CAD build for the part. Positions are in the model's coordinates, mm. Face numbers are marked on the shaded views. A direction names the side the tool comes from. Coordinates: 2 decimals unless noted, no trailing zeros. Order: outer loops, then holes, each group sorted by start corner. A loop starts at its lowest first (then second) coordinate and runs counter-clockwise, first axis right, second up. Notation, with made-up numbers: M -22.75,77.25 L 23.25,77.25 A16 ccw 23.25,87.25 Z; hole C 69,73 d1. An arc over 180 degrees is marked long. One line per item, written item: value.
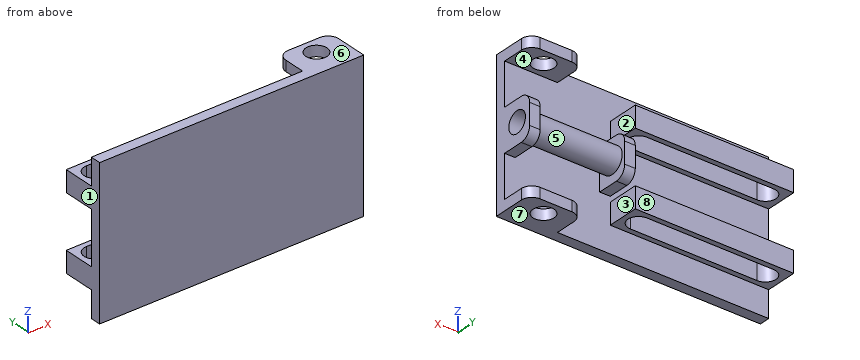
from build123d import *

# Parameters (mm, degrees)
SKETCH1_W           = 250
SKETCH1_H           = 140
BOSS_EXTRUDE1_DEPTH = 10
SKETCH2_W           = 150
SKETCH2_H           = 20
SKETCH2_W_2         = 50
BOSS_EXTRUDE2_DEPTH = 30
CUT_EXTRUDE1_DEPTH  = 120
SKETCH4_R           = 10
CUT_EXTRUDE2_DEPTH  = 150
SKETCH6_W           = 10
SKETCH6_H           = 40
CUT_EXTRUDE4_DEPTH  = 150
SKETCH7_R           = 10
CUT_EXTRUDE5_DEPTH  = 150
SKETCH8_R           = 12
SKETCH8_R_2         = 10
BOSS_EXTRUDE3_DEPTH = 80
SKETCH9_W           = 40
SKETCH9_H           = 30
SKETCH9_R           = 10
BOSS_EXTRUDE4_DEPTH = 10
FILLET1_R           = 10
FILLET2_R           = 10
FILLET3_R           = 10
SKETCH13_W          = 50
SKETCH13_H          = 25
SKETCH13_H_2        = 22.244291656
CUT_EXTRUDE6_DEPTH  = 40


with BuildPart() as part:
    # Sketch1 → Boss-Extrude1 (new body)
    with BuildSketch(Plane(origin=(0, 0, 0), x_dir=(1, 0, 0), z_dir=(0, 1, 0))):
        Rectangle(SKETCH1_W, SKETCH1_H)
    extrude(amount=BOSS_EXTRUDE1_DEPTH)

    # Sketch2 → Boss-Extrude2 (add)
    with BuildSketch(Plane(origin=(0, 10, 0), x_dir=(1, 0, 0), z_dir=(0, 1, 0))):
        with Locations((-50, 35)):
            Rectangle(SKETCH2_W, SKETCH2_H)
        with Locations((-50, -35)):
            Rectangle(SKETCH2_W, SKETCH2_H)
        Polygon((125, -20), (125, 0), (125, 20), (105, 20), (105, -20), align=None)
        with Locations((100, 60)):
            Rectangle(SKETCH2_W_2, SKETCH2_H)
        with Locations((100, -60)):
            Rectangle(SKETCH2_W_2, SKETCH2_H)
    extrude(amount=BOSS_EXTRUDE2_DEPTH)

    # Sketch3 → Cut-Extrude1 (cut)
    with BuildSketch(Plane.XY.offset(45)):
        with BuildLine():
            Line((10, 35), (-110, 35))
            ThreePointArc((-110, 35), (-120, 25), (-110, 15))
            Line((-110, 15), (10, 15))
            ThreePointArc((10, 15), (20, 25), (10, 35))
        make_face()
    extrude(amount=-CUT_EXTRUDE1_DEPTH, mode=Mode.SUBTRACT)

    # Sketch4 → Cut-Extrude2 (cut)
    with BuildSketch(Plane.XY.offset(70)):
        with Locations((100, 25)):
            Circle(SKETCH4_R)
    extrude(amount=-CUT_EXTRUDE2_DEPTH, mode=Mode.SUBTRACT)

    # Sketch6 → Cut-Extrude4 (cut)
    with BuildSketch(Plane(origin=(0, 10, 0), x_dir=(1, 0, 0), z_dir=(0, 1, 0))):
        with Locations((110, 0)):
            Rectangle(SKETCH6_W, SKETCH6_H)
    extrude(amount=CUT_EXTRUDE4_DEPTH, mode=Mode.SUBTRACT)

    # Sketch7 → Cut-Extrude5 (cut)
    with BuildSketch(Plane(origin=(125, 0, 0), x_dir=(0, 0, -1), z_dir=(1, 0, 0))):
        with Locations((0, 25)):
            Circle(SKETCH7_R)
    extrude(amount=-CUT_EXTRUDE5_DEPTH, mode=Mode.SUBTRACT)

    # Sketch8 → Boss-Extrude3 (add)
    with BuildSketch(Plane.ZY.offset(-115)):
        with Locations((0, 25)):
            Circle(SKETCH8_R)
        with Locations(Location((0, 25, 0), (0, 0, 180))):
            Circle(SKETCH8_R_2, mode=Mode.SUBTRACT)
    extrude(amount=BOSS_EXTRUDE3_DEPTH)

    # Sketch9 → Boss-Extrude4 (add)
    with BuildSketch(Plane.ZY.offset(-35)):
        with Locations((0, 25)):
            Rectangle(SKETCH9_W, SKETCH9_H)
        with Locations(Location((0, 25, 0), (0, 0, 180))):
            Circle(SKETCH9_R, mode=Mode.SUBTRACT)
    extrude(amount=BOSS_EXTRUDE4_DEPTH)

    # Fillet1
    fillet1_edges = [part.edges().sort_by_distance(p)[0] for p in [
        (30, 40, 20),
        (30, 40, -20),
    ]]
    fillet(fillet1_edges, radius=FILLET1_R)

    # Fillet2
    fillet2_edges = [part.edges().sort_by_distance(p)[0] for p in [
        (120, 40, 20),
        (120, 40, -20),
    ]]
    fillet(fillet2_edges, radius=FILLET2_R)

    # Fillet3
    fillet3_edges = [part.edges().sort_by_distance(p)[0] for p in [
        (75, 40, -60),
        (125, 40, -60),
        (75, 40, 60),
        (125, 40, 60),
    ]]
    fillet(fillet3_edges, radius=FILLET3_R)

    # Sketch13 → Cut-Extrude6 (cut)
    with BuildSketch(Plane(origin=(0, 10, 0), x_dir=(1, 0, 0), z_dir=(0, 1, 0))):
        with Locations((100, 47.5)):
            Rectangle(SKETCH13_W, SKETCH13_H)
        with Locations((100, -48.877854172)):
            Rectangle(SKETCH13_W, SKETCH13_H_2)
    extrude(amount=CUT_EXTRUDE6_DEPTH, mode=Mode.SUBTRACT)


solid = part.part
Q1. Slice it at D-D (y = 25). Give the number of separate pieces and of enclosed holes in the cut face, plus the area to 3 significant figures.
Recorded:
separate pieces: 10
enclosed holes: 0
area: 1,720 mm^2
Q2. Pin check, flat tips, straight feed: pin 1 Ø8 at (y, z) = (19.5, -65.5) entering from -X; pin 2 Ø8 at (x, z) = (-32, -3.5) entering from +Y; pin 3 Ø16 at (y, z) = (25, -35) entering from +X; pin 4 Ø9 at (x, y) = (-62.5, 22) entering from -Z. Stop position of each tip, or through.
Recorded:
pin 1: stops at x = 75
pin 2: stops at y = 10
pin 3: stops at x = 25
pin 4: passes through
Q3. Slice it at C-C (x = -100.5). List the corners of the cut face in (y, z), plus the area to 3 significant figures.
Recorded:
outline: M 0,-70 L 10,-70 L 10,-45 L 15,-45 L 15,-25 L 10,-25 L 10,25 L 15,25 L 15,45 L 10,45 L 10,70 L 0,70 Z; M 35,-45 L 40,-45 L 40,-25 L 35,-25 Z; M 35,25 L 40,25 L 40,45 L 35,45 Z
area: 1,800 mm^2
Q4. Mould opens along Z. For the marked faces 5, 6, 7 and 8 say: released by +Z, released by -Z, zero draft, split by the parting line, or undercut.
Recorded:
face 5: undercut
face 6: released by +Z
face 7: released by -Z
face 8: zero draft
Q5. Which spindle directions (+Z, -Z, +X, -X, +Y, -Y) get a long thin tool onto all of the face, cutting with end or side? Do the marked faces 1, 2, 3 and 4. Say none if no direction does.
Recorded:
face 1: +Z, -Z, -X, +Y, -Y
face 2: +Z, +X, +Y
face 3: -Z, +X, +Y
face 4: +X, -X, +Y
Q6. Slice it at A-A (z = 0). List the corners of the cut face in (x, y).
Recorded:
outline: M -125,0 L 125,0 L 125,15 L 25,15 L 25,10 L -125,10 Z; M 25,35 L 125,35 L 125,40 L 115,40 L 115,37 L 35,37 L 35,40 L 25,40 Z; hole M 35,10 L 115,10 L 115,13 L 35,13 Z
Q7. Drill centre lines: line 1 along Z through (x, y) = (-106.5, 13); line 2 along X through (y, z) = (15, -15.5); line 3 along Z through (x, y) = (81, 18.5). Where is each one in solid material? Low to high.
Recorded:
line 1: z = -45 to -25, 25 to 45
line 2: x = 25 to 35, 115 to 125
line 3: z = -70 to -60, -10.09 to -7.6, 7.6 to 10.09, 60 to 70
Q8. Slice it at B-B (x = 100). List the corners of the cut face in (y, z).
Recorded:
outline: M 0,-70 L 15,-70 L 15,-60 L 10,-60 L 10,60 L 15,60 L 15,70 L 0,70 Z; C 25,0 d24; M 35,-70 L 40,-70 L 40,-60 L 35,-60 Z; M 35,60 L 40,60 L 40,70 L 35,70 Z; hole C 25,0 d20
